Work out the finished part from the listing and answer in its coordinate system (mm). A direction names the side the tool comes from. Give positions to 0.01 mm unless a question says otherwise; leave off trailing zeros. Order: outer loops, then holes, each group sorted by start corner. A loop starts at its lowest first (then second) coordinate and runs counter-clockwise, first axis right, second up. Notation, with made-up numbers: (28, 74) - (38, 74) arc R10 cw to (38, 90) - close; hole circle Ø4 at (-17.75, -37). An arc over 180 degrees is marked (long way). Write each question's results on one line, items separated by ' | '.
from build123d import *

# Parameters (mm, degrees)
F1_DEPTH  = 16
F2_R      = 3
F3_DEPTH  = 20
F5_DEPTH  = 6
F7_DEPTH  = 3
F8_R      = 3
F9_DEPTH  = 3
F10_DEPTH = 20


with BuildPart() as f1:
    # F0 (on Front) → F1 (new body)
    with BuildSketch(Plane.XZ):
        Polygon((3, 72), (-3, 72), (-3, 0), (0, 0), (3, 0), align=None)
        Polygon((0, 0), (-3, 0), (-10, -8), (-10, -32), (-14, -40), (-14, -75), (-10, -83), (-10, -89), (-7, -89), (-7, -83), (-11, -75), (-11, -40), (-7, -32), (-7, -8), align=None)
        Polygon((10, -8), (3, 0), (0, 0), (7, -8), (7, -32), (11, -40), (11, -75), (7, -83), (7, -89), (10, -89), (10, -83), (14, -75), (14, -40), (10, -32), align=None)
    extrude(amount=F1_DEPTH)

    # F2 (on face) → F3 (cut)
    with BuildSketch(Plane(origin=(-10, 0, 0), x_dir=(0, -1, 0), z_dir=(-1, 0, 0))):
        with Locations((8, -25)):
            Circle(F2_R)
    extrude(amount=-F3_DEPTH, mode=Mode.SUBTRACT)

    # F4 (on face) → F5 (join)
    with BuildSketch(Plane(origin=(-3, 0, 0), x_dir=(0, -1, 0), z_dir=(-1, 0, 0))):
        with BuildLine():
            Line((0, 72), (16, 72))
            ThreePointArc((16, 72), (8, 80), (0, 72))
        make_face()
    extrude(amount=-F5_DEPTH)

    # F6 (on face) → F7 (join)
    with BuildSketch(Plane(origin=(-10, 0, 0), x_dir=(0, -1, 0), z_dir=(-1, 0, 0))):
        with BuildLine():
            Line((16, -89), (0, -89))
            ThreePointArc((0, -89), (8, -97), (16, -89))
        make_face()
    extrude(amount=-F7_DEPTH)

    # F8 (on face) → F9 (join)
    with BuildSketch(Plane.YZ.offset(10)):
        with Locations((-8, -89)):
            Circle(F8_R)
        with BuildLine():
            Line((-11, -89), (-16, -89))
            ThreePointArc((-16, -89), (-8, -97), (0, -89))
            Line((0, -89), (-5, -89))
            ThreePointArc((-5, -89), (-8, -92), (-11, -89))
        make_face()
    extrude(amount=-F9_DEPTH)

    # F8 (on face) → F10 (cut)
    with BuildSketch(Plane.YZ.offset(10)):
        with Locations((-8, -89)):
            Circle(F8_R)
    extrude(amount=-F10_DEPTH, mode=Mode.SUBTRACT)


solid = f1.part
1. Determine the mould class of faces 1 (the face through (-10, -8, -20)), 2 (the face through (-7.3, 0, -14.1)), 3 (the face through (-9, -8, -79)) for opening direction X: +X half, -X half, draft (parallel to the pull), parting line (faces both ways), or undercut.
Answer list:
face 1: -X half | face 2: draft | face 3: undercut
2. Given P1, Ø1, axis at x = -4, y = -10.5, coming from the +Z side; P2, Ø12, axis at x = -10, z = 14.5, coming from the +Y side; P3, Ø7, axis at y = -11, z = -89, coming from the +X side; P4, Ø8, axis at y = -8, z = -89, coming from the -X side, each flat-ended and moving along its own axis, determine where each tip first touches the part or whether it passes through.
Answer list:
P1: z = -0.57 | P2: through | P3: x = 10 | P4: x = -10
3. Straight lines are drawn through the part: line 1 (Z direction, x = -9.25, y = -8); line 2 (X direction, y = -14, z = -30); line 3 (X direction, y = -3.25, z = 38). For each, find the intervals that lie inside material, in ascending order. Write a range as [from, to].
Answer list:
line 1: [-97, -92], [-86, -78.5], [-36.5, -28], [-22, -7.14] | line 2: [-10, -7], [7, 10] | line 3: [-3, 3]
4. A tool of negligible diameter and unlimited length cuts with its end or side. For faces 4 (the face through (-11, -8, -58)), 5 (the face through (-7, -11, -90)), 6 (the face through (10, -5, -90)), from which of +Z, -Z, +X, -X, +Y, -Y can it reach the whole face along a straight path? Write none if from no direction.
Answer list:
face 4: +Y, -Y | face 5: -Z, +Y, -Y | face 6: -Z, +X, +Y, -Y
5. A cutting plane is placed at B-B, the plane z = -73. Write down the section's boundary in (x, y), then the cut area to 3 significant figures.
Answer list:
outline: (-14, -16) - (-11, -16) - (-11, 0) - (-14, 0) - close; (11, -16) - (14, -16) - (14, 0) - (11, 0) - close | area: 96.0 mm^2
6. A cutting plane is placed at A-A, the plane x = -8.5. Write down the section's boundary in (y, z).
Answer list:
outline: (-16, -89) arc R8 ccw to (0, -89) - (0, -80) - (-16, -80) - close; (-16, -35) - (0, -35) - (0, -6.29) - (-16, -6.29) - close; hole circle Ø6 at (-8, -89); hole circle Ø6 at (-8, -25)
7. A cutting plane is placed at D-D, the plane z = 57. Write down the section's boundary in (x, y), then the cut area to 3 significant figures.
Answer list:
outline: (-3, -16) - (3, -16) - (3, 0) - (-3, 0) - close | area: 96.0 mm^2
